Check sheet for the modelled part. Datum: model origin and axes. Units: mm. Face numbers are marked on the shaded views. A direction names the side the tool comes from. Give positions to 0.01 mm unless a question says otherwise; leave off trailing zeros. Order: outer loops, then holes, each group sorted by start corner. A loop starts at its lowest first (then second) coordinate and runs counter-clockwise, first axis right, second up.
```python
from build123d import *

# Parameters (mm, degrees)
SKETCH1_R           = 3.5
SKETCH1_R_2         = 2.3
BOSS_EXTRUDE1_DEPTH = 2.5
BOSS_EXTRUDE2_START = -2
SKETCH1_3_R         = 3.5
SKETCH1_3_R_2       = 2.3
BOSS_EXTRUDE2_DEPTH = 2
BOSS_EXTRUDE3_START = -1
SKETCH2_R           = 2.3
SKETCH2_R_2         = 1.5
BOSS_EXTRUDE3_DEPTH = 1
SKETCH3_R           = 0.6
CUT_EXTRUDE1_DEPTH  = 10


with BuildPart() as part:
    # Sketch1 → Boss-Extrude1 (new body)
    with BuildSketch(Plane(origin=(0, 0, 0), x_dir=(1, 0, 0), z_dir=(0, 1, 0))):
        with Locations(Location((0, 0, 0), (0, 0, 270))):
            Circle(SKETCH1_R)
        with Locations(Location((0, 0, 0), (0, 0, 270))):
            Circle(SKETCH1_R_2, mode=Mode.SUBTRACT)
    extrude(amount=BOSS_EXTRUDE1_DEPTH)

    # Sketch1_3 → Boss-Extrude2 (add)
    # profile 1 of 2: a face of its own
    with BuildSketch(Plane(origin=(0, 0, 0), x_dir=(1, 0, 0), z_dir=(0, 1, 0)).offset(BOSS_EXTRUDE2_START)):
        with Locations(Location((0, 0, 0), (0, 0, 42.557900428))):
            Circle(SKETCH1_3_R)
        with Locations(Location((0, 0, 0), (0, 0, 270))):
            Circle(SKETCH1_3_R_2, mode=Mode.SUBTRACT)
    # profile 2 of 2: a face of its own
    with BuildSketch(Plane(origin=(0, 0, 0), x_dir=(1, 0, 0), z_dir=(0, 1, 0)).offset(BOSS_EXTRUDE2_START)):
        with BuildLine():
            ThreePointArc((14.25, -1.75), (16, 0), (14.25, 1.75))
            Line((14.25, 1.75), (2.578079842, 2.367172221))
            ThreePointArc((2.578079842, 2.367172221), (3.261386166, 1.270181198), (3.5, 0))
            ThreePointArc((3.5, 0), (3.261386166, -1.270181198), (2.578079842, -2.367172221))
            Line((2.578079842, -2.367172221), (14.25, -1.75))
        make_face()
    extrude(amount=BOSS_EXTRUDE2_DEPTH)

    # Sketch2 → Boss-Extrude3 (add)
    with BuildSketch(Plane(origin=(0, 0, 0), x_dir=(1, 0, 0), z_dir=(0, 1, 0)).offset(BOSS_EXTRUDE3_START)):
        with Locations(Location((0, 0, 0), (0, 0, 270))):
            Circle(SKETCH2_R)
        with Locations(Location((0, 0, 0), (0, 0, 270))):
            Circle(SKETCH2_R_2, mode=Mode.SUBTRACT)
    extrude(amount=BOSS_EXTRUDE3_DEPTH)

    # Sketch3 → Cut-Extrude1 (cut)
    with BuildSketch(Plane.XZ.offset(2)):
        with Locations(Location((9, 0, 0), (0, 0, 270))):
            Circle(SKETCH3_R)
    extrude(amount=-CUT_EXTRUDE1_DEPTH, mode=Mode.SUBTRACT)


solid = part.part
```
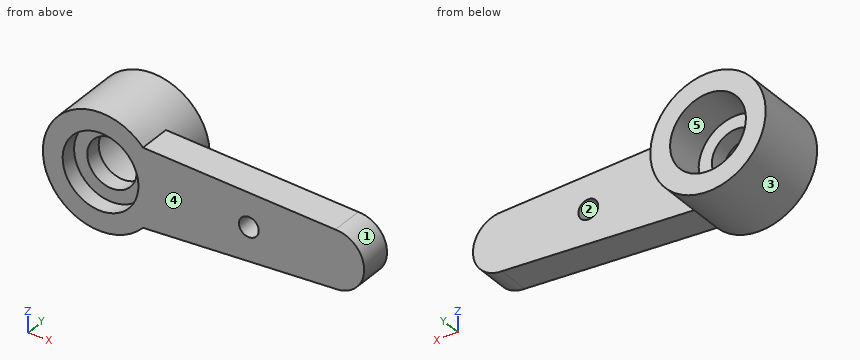
Q1. Sectioned sample at D-D, the plane x = -1.25. Record the cut outline in (y, z), plus the area to 3 significant figures.
Q2. Sectioned sample at B-B, the plane x = 8.75. Record the cut outline in (y, z).
Q3. Draft check along X on the marked faces 1, 2 and 3. Enter one of: pulls with the +X half, pulls with the -X half, needs draft (parallel to the pull), parting line crosses it, or undercut.
Q4. Go/stop test with flat-tipped pins: P1, Ø2, axis at y = -1.5, z = -3, coming from the -X side; P2, Ø1.8, axis at x = 0, z = 0, coming from the +Y side; P3, Ø3, axis at x = 11.5, z = 3, coming from the +Y side; P4, Ø4, axis at x = 0, z = 0, coming from the -Y side. Record where each tip stops, or that it passes through.
Q5. Sectioned sample at C-C, the plane y = -0.5. Record the cut outline in (x, z), plus the area to 3 significant figures.
Q6. Tool access check on the marked faces 4 and 5. Record the directions out of +Z, -Z, +X, -X, +Y, -Y that give a thin tool (end or side, any length) a straight path to the whole face; none if there is none.
Q7. Material ranges on line 1 (X direction, y = -0.5, z = 0); line 2 (X direction, y = -1.65, z = 0); line 3 (X direction, y = 1.8, z = 0), recorded low to high.
Filled in:
1. outline: (-2, -3.27) - (2.5, -3.27) - (2.5, -1.93) - (0, -1.93) - (0, -0.83) - (-1, -0.83) - (-1, -1.93) - (-2, -1.93) - close; (-2, 1.93) - (-1, 1.93) - (-1, 0.83) - (0, 0.83) - (0, 1.93) - (2.5, 1.93) - (2.5, 3.27) - (-2, 3.27) - close
1. area: 14.2 mm2
2. outline: (-2, -2.04) - (0, -2.04) - (0, -0.55) - (-2, -0.55) - close; (-2, 0.55) - (0, 0.55) - (0, 2.04) - (-2, 2.04) - close
3. face 1: pulls with the +X half
3. face 2: undercut
3. face 3: parting line crosses it
4. P1: stops at x = -2.87
4. P2: passes through
4. P3: stops at y = 0
4. P4: stops at y = -1
5. outline: (2.58, -2.37) - (14.25, -1.75) arc R1.75 ccw to (14.25, 1.75) - (2.58, 2.37) arc R3.5 ccw (long way) to start; hole circle Ø3 at (0, 0); hole circle Ø1.2 at (9, 0)
5. area: 80.2 mm2
6. face 4: +Z, -Z, +X, -X, -Y
6. face 5: +Y
7. line 1: x = -3.5 to -1.5, 1.5 to 8.4, 9.6 to 16
7. line 2: x = -3.5 to -2.3, 2.3 to 8.4, 9.6 to 16
7. line 3: x = -3.5 to -2.3, 2.3 to 3.5
